Autodesk Inventor part; units mm, degrees
ref_plane "YZ Plane" through (0, 0, 0) normal (1, 0, 0) x (0, 1, 0)
ref_plane "XZ Plane" through (0, 0, 0) normal (0, 1, 0) x (-1, 0, 0)
ref_plane "XY Plane" through (0, 0, 0) normal (0, 0, 1) x (1, 0, 0)
sketch "Sketch1" plane through (0, 0, 0) normal (0, 0, 1) x (1, 0, 0)
  circle A0 centre (-414.4261, -56.251) radius 4.7625
  point P0 (0, 0)
  dimension "d0" = 9.525
extrude "Extrusion1" add sketch "Sketch1" against normal blind 165.1
sketch "Sketch2" plane through (-414.4261, -56.251, 0) normal (0, 0, 1) x (1, 0, 0)
  circle A0 centre (0, 0) radius 4.7625
  line L0 (-8.2489, 0) -> (-4.1244, 7.1437)
  line L1 (-4.1244, 7.1437) -> (4.1244, 7.1438)
  line L2 (4.1244, 7.1438) -> (8.2489, 0)
  line L3 (8.2489, 0) -> (4.1244, -7.1437)
  line L4 (4.1244, -7.1437) -> (-4.1244, -7.1438)
  line L5 (-4.1244, -7.1438) -> (-8.2489, 0)
  point P0 (414.4261, 56.251)
  dimension "d3" = 14.2875
extrude "Extrusion2" add sketch "Sketch2" along normal blind 3.175 contours A0 | L0 L1 L2 L3 L4 L5
thread "Thread1"
chamfer "Chamfer1" distance 0.508 angle 45 1 edges at (-419.1886, -56.251, -165.1)
properties part number "38-16 hexbolt x6500" material "Steel"
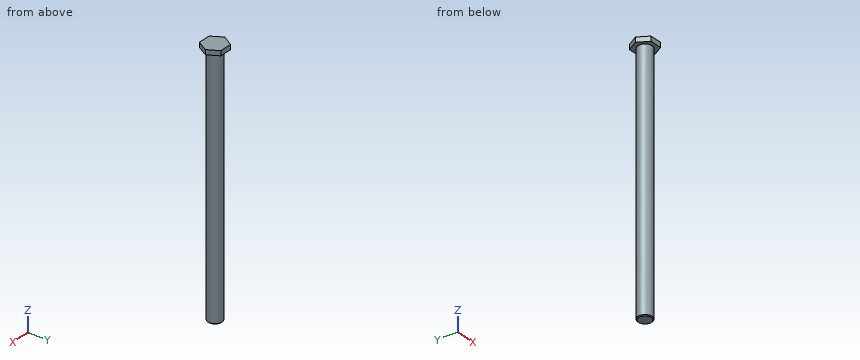
Build history of the part. All positions in model axes, mm. Coordinates: 2 decimals unless noted, no trailing zeros. Order: outer loops, then holes, each group sorted by start corner. A loop starts at its lowest first (then second) coordinate and runs counter-clockwise, first axis right, second up. Notation, with made-up numbers: (-24.75, -22) -> (-7.75, -22) arc R16 cw to (-7.75, 6) -> close; hole circle Ø4 at (-11, 27.25). An arc over 180 degrees is marked (long way). Answer in a Markdown table with one row per item. Add a question column.
Q1. Band-saw the part on A-A, the plane z = -142. List the corners of the cut face in (x, y) (1 decimal), then the cut area to 3 significant figures.
Q2. Band-saw the part on B-B, the plane x = -408. List the corners of the cut face in (y, z) (3 decimals), then the cut area to 3 significant figures.
Q3. Drop flat-ended pins along their axis: pin 1 (1 mm diameter, centred on x = -418, z = -109, fed in from -Y); pin 2 (4 mm diameter, centred on y = -52, z = -125, fed in from -X); pin 3 (4 mm diameter, centred on x = -420.5, z = -83, fed in from -Y). Give the stop position or say it passes through.
Q4. Wall check: line 1 along Z through (x, y) = (-420.5, -57.5) (3 decimals); line 2 along X through (y, z) = (-56, -104); line 3 along Y through (x, z) = (-416.5, -131). Give the ranges that are in metal, low to high. Write a range as [from, to].
Answers follow:
| question | item | result |
|---|---|---|
| 1 | outline | circle Ø9.5 at (-414.4, -56.3) |
| 1 | area | 71.3 mm^2 |
| 2 | outline | (-59.408, 0) -> (-53.094, 0) -> (-53.094, 3.175) -> (-59.408, 3.175) -> close |
| 2 | area | 20.0 mm^2 |
| 3 | pin 1 | y = -59.89 |
| 3 | pin 2 | x = -418.62 |
| 3 | pin 3 | y = -58.72 |
| 4 | line 1 | [0, 3.175] |
| 4 | line 2 | [-419.18, -409.67] |
| 4 | line 3 | [-60.54, -51.96] |
